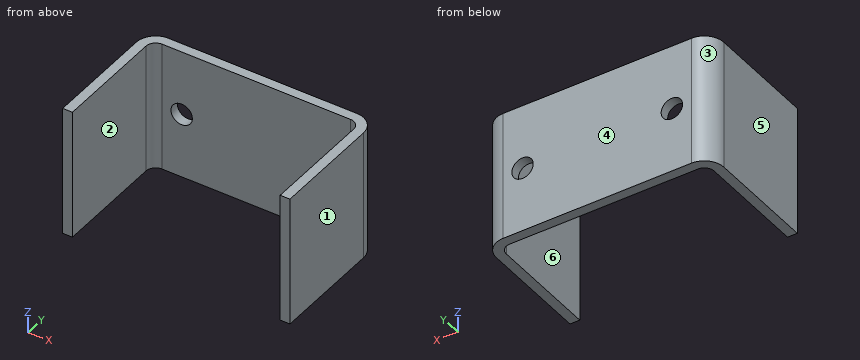
```python
from build123d import *

# Parameters (mm, degrees)
SM_BASE_FLANGE_1_DEPTH  = 20
HOLE_WIZARD_6_6_6_6_1_D = 6.6


# Sheet-metal steps are written as plain solids
with BuildPart() as part:
    # Sketch 1 → Базовая кромка1 (new, symmetric)
    with BuildSketch(Plane.XY):
        with BuildLine():
            Line((0, 0), (0, 34))
            ThreePointArc((0, 34), (1.757359313, 38.242640687), (6, 40))
            Line((6, 40), (64, 40))
            ThreePointArc((64, 40), (68.242640687, 38.242640687), (70, 34))
            Line((70, 34), (70, 0))
            Line((70, 0), (67, 0))
            Line((67, 0), (67, 34))
            ThreePointArc((67, 34), (66.121320344, 36.121320344), (64, 37))
            Line((64, 37), (6, 37))
            ThreePointArc((6, 37), (3.878679656, 36.121320344), (3, 34))
            Line((3, 34), (3, 0))
            Line((3, 0), (0, 0))
        make_face()
    extrude(amount=SM_BASE_FLANGE_1_DEPTH, both=True)

    # Диаметр отверстия Ø6.6 (6.6)1 (through all)
    with Locations(Plane(origin=(0, 40, 0), x_dir=(1, 0, 0), z_dir=(0, 1, 0))):
        with Locations((12, 0), (58, 0)):
            Hole(HOLE_WIZARD_6_6_6_6_1_D / 2)


solid = part.part
```
Model file for the job. Use its own axes, mm. Face numbers are marked on the shaded views. A direction names the side the tool comes from. Give positions to 0.01 mm unless a question says otherwise; leave off trailing zeros. Write each loop counter-clockwise with the first axis right and the second up, starting at its lowest first coordinate (ties: lowest second). Pieces come first, ordered by that corner, then holes. Notation, with made-up numbers: (62.25, 79) - (101.25, 79) arc R28 ccw to (101.25, 102) - close; hole circle Ø3 at (-31.75, -32.75). An arc over 180 degrees is marked (long way). One line per question, with ' | ' between items. Start each with the question number.
(1) Two-plate mould, pull along X, no slides. Class the marked faces 1, 2, 3 and 4: +X half, -X half, draft (parallel to the pull), parting line (faces both ways), or undercut.
(2) Slice it at C-C on z = 0. Write the cut outline in (x, y).
(3) 3-axis set-ups, long thin cutter, end or side, ignore diameter. For the marked faces 5 and 6: which of +Z, -Z, +X, -X, +Y, -Y reach the whole face in a straight line?
(4) Slice it at D-D on x = 43. Write the cut outline in (y, z).
(5) Pin check, flat tips, straight feed: P1, Ø12, axis at x = 25, z = 3, coming from the -Y side; P2, Ø1, axis at y = 35, z = -5.5, coming from the +X side. Stop position of each tip, or through.
(6) Wall check: line 1 along X through (y, z) = (6, 2.5); line 2 along Z through (x, y) = (58, 38.95); line 3 along Y through (x, z) = (20, -4.5). Give the ranges that are in metal, low to high. Write a range as from..to.
(7) Slice it at A-A on x = 12. Write the cut outline in (y, z), plus the area to 3 significant figures.
(8) Slice it at B-B on y = 20. Write the cut outline in (x, z), plus the area to 3 significant figures.
Results below:
1) face 1: +X half | face 2: undercut | face 3: -X half | face 4: draft
2) outline: (0, 0) - (3, 0) - (3, 34) arc R3 cw to (6, 37) - (8.7, 37) - (8.7, 40) - (6, 40) arc R6 ccw to (0, 34) - close; (15.3, 37) - (54.7, 37) - (54.7, 40) - (15.3, 40) - close; (61.3, 37) - (64, 37) arc R3 cw to (67, 34) - (67, 0) - (70, 0) - (70, 34) arc R6 ccw to (64, 40) - (61.3, 40) - close
3) face 5: +Z, -Z, -X, +Y, -Y | face 6: +Z, -Z, -Y
4) outline: (37, -20) - (40, -20) - (40, 20) - (37, 20) - close
5) P1: y = 37 | P2: x = 69.98
6) line 1: 0..3, 67..70 | line 2: -20..-3.3, 3.3..20 | line 3: 37..40
7) outline: (37, -20) - (40, -20) - (40, -3.3) - (37, -3.3) - close; (37, 3.3) - (40, 3.3) - (40, 20) - (37, 20) - close | area: 100 mm^2
8) outline: (0, -20) - (3, -20) - (3, 20) - (0, 20) - close; (67, -20) - (70, -20) - (70, 20) - (67, 20) - close | area: 240 mm^2
